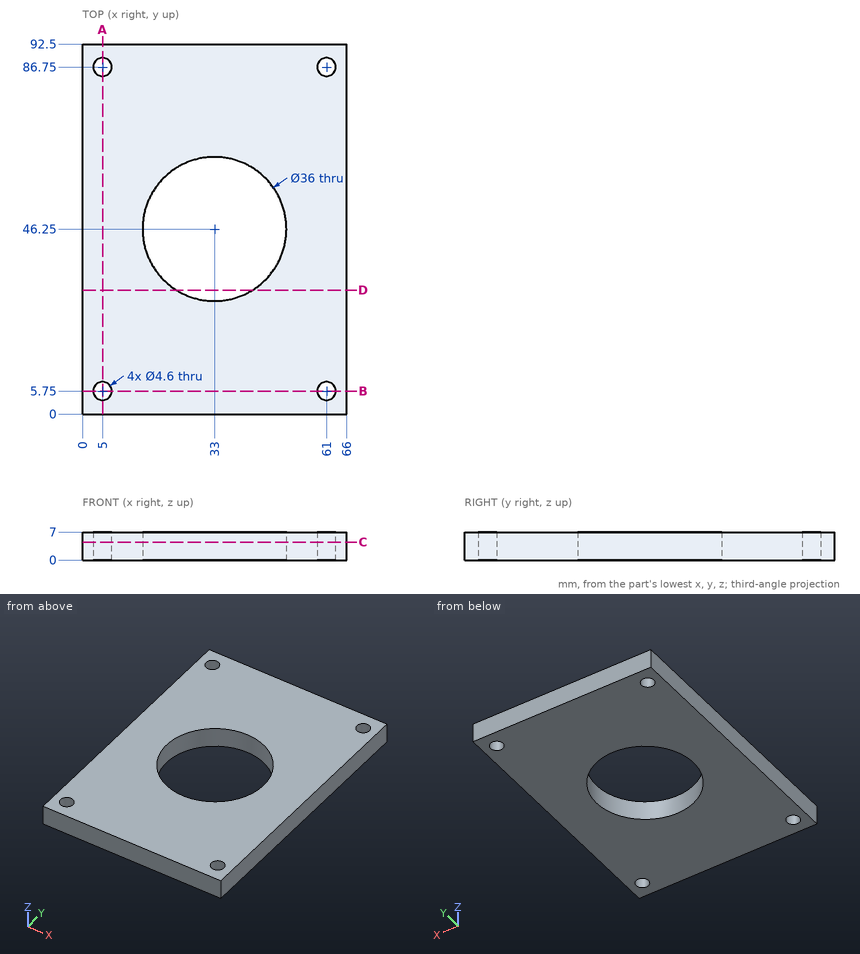
Print and shaded views of the part. All mm, measured from the part's lowest x, y and z. Round coordinates to 2 decimals unless told otherwise and drop trailing zeros. Loops run counter-clockwise (first coordinate to the right, second up) from the corner with the lowest first, then second, coordinate; pieces in that order, holes last. Notation, with made-up numbers: (-32.5, -32.5) -> (14.5, -32.5) arc R22 cw to (14.5, -10.5) -> close; hole circle Ø8 at (-9, 72). An arc over 180 degrees is marked (long way). Use CSV: the item, a comma, the result in double quotes. Start each with the question number.
1) Cut at B-B, the plane y = 5.75. Write the cut outline in (x, z), plus the area to 3 significant figures.
2) Cut at A-A, the plane x = 5. Write the cut outline in (y, z), plus the area to 3 significant figures.
3) Cut at D-D, the plane y = 31. Write the cut outline in (x, z), plus the area to 3 significant figures.
4) Drop flat-ended pins along their axis: P1, Ø5.5, axis at x = 5, y = 86.75, coming from the -Z side; P2, Ø3.5, axis at x = 5, y = 5.75, coming from the -Z side. Give the stop position or say it passes through.
5) Wall check: L1, parallel to Y at x = 61, z = 4.25; L2, parallel to X at y = 86.75, z = 1.5; L3, parallel to Y at x = 6.5, z = 5. Give the ranges that are in metal, low to high. Write a range as [from, to].
6) Cut at C-C, the plane z = 4.5. Write the cut outline in (x, y).
Determined:
1,outline,"(0, 0) -> (2.7, 0) -> (2.7, 7) -> (0, 7) -> close; (7.3, 0) -> (58.7, 0) -> (58.7, 7) -> (7.3, 7) -> close; (63.3, 0) -> (66, 0) -> (66, 7) -> (63.3, 7) -> close"
1,area,"398 mm2"
2,outline,"(0, 0) -> (3.45, 0) -> (3.45, 7) -> (0, 7) -> close; (8.05, 0) -> (84.45, 0) -> (84.45, 7) -> (8.05, 7) -> close; (89.05, 0) -> (92.5, 0) -> (92.5, 7) -> (89.05, 7) -> close"
2,area,"583 mm2"
3,outline,"(0, 0) -> (23.44, 0) -> (23.44, 7) -> (0, 7) -> close; (42.56, 0) -> (66, 0) -> (66, 7) -> (42.56, 7) -> close"
3,area,"328 mm2"
4,P1,"stops at z = 0"
4,P2,"passes through"
5,L1,"y = [0, 3.45], [8.05, 84.45], [89.05, 92.5]"
5,L2,"x = [0, 2.7], [7.3, 58.7], [63.3, 66]"
5,L3,"y = [0, 4.01], [7.49, 85.01], [88.49, 92.5]"
6,outline,"(0, 0) -> (66, 0) -> (66, 92.5) -> (0, 92.5) -> close; hole circle Ø4.6 at (5, 5.75); hole circle Ø4.6 at (5, 86.75); hole circle Ø36 at (33, 46.25); hole circle Ø4.6 at (61, 5.75); hole circle Ø4.6 at (61, 86.75)"
